Print and shaded views of the part. All mm, measured from the part's lowest x, y and z. A direction names the side the tool comes from. Round coordinates to 2 decimals unless told otherwise and drop trailing zeros. Order: outer loops, then holes, each group sorted by start corner. A loop starts at its lowest first (then second) coordinate and runs counter-clockwise, first axis right, second up. Notation, with made-up numbers: (34.5, 59) -> (70.5, 59) arc R9 cw to (70.5, 76) -> close; hole circle Ø5 at (-0.5, -36). An arc over 180 degrees is marked (long way). Answer as CSV lines item,"result".
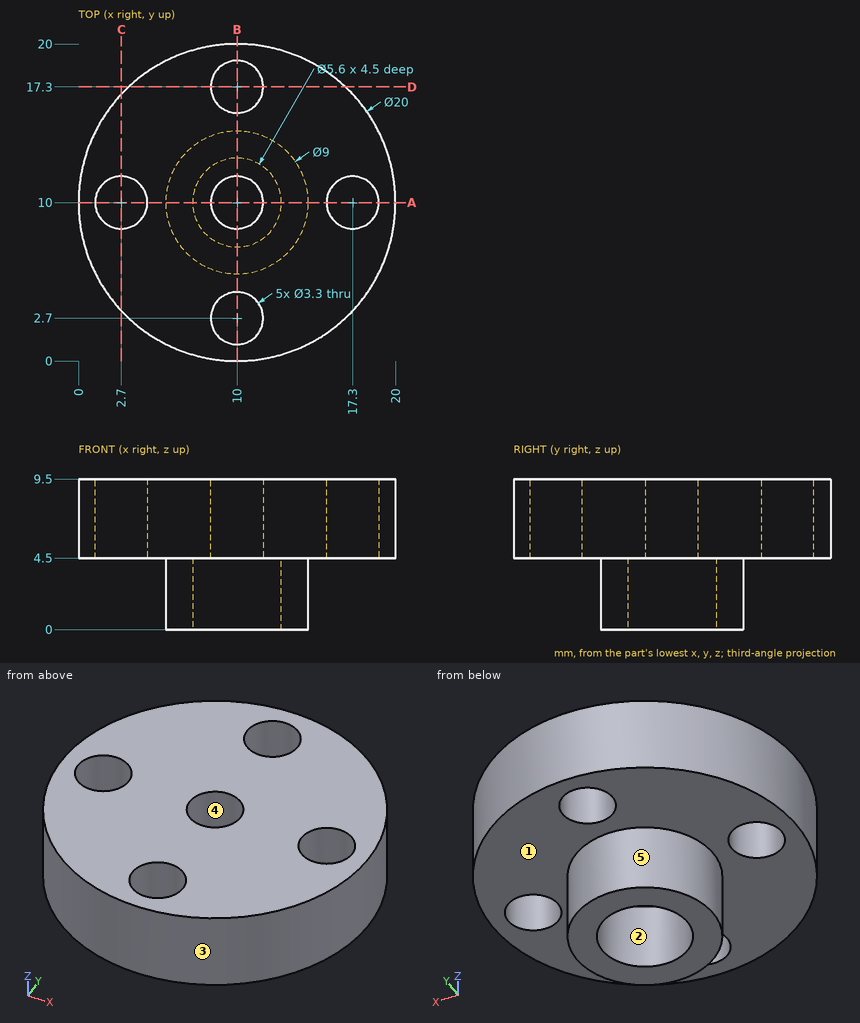
Q1. Tool access for the marked faces 4 and 5: list every direction of +Z, -Z, +X, -X, +Y, -Y with a clear straight run to the whole face (end or side of a thin tool).
Checks:
face 4,"+Z, -Z"
face 5,"-Z"
Q2. Mould opens along X. For the marked faces 1, 2 and 3 say: +X half, -X half, draft (parallel to the pull), parting line (faces both ways), or undercut.
Checks:
face 1,"draft"
face 2,"undercut"
face 3,"parting line"
Q3. Saw through at C-C (x = 2.7). Write the cut outline in (y, z), plus the area to 3 significant figures.
Checks:
outline,"(3.17, 4.5) -> (8.35, 4.5) -> (8.35, 9.5) -> (3.17, 9.5) -> close; (11.65, 4.5) -> (16.83, 4.5) -> (16.83, 9.5) -> (11.65, 9.5) -> close"
area,"51.8 mm²"
Q4. Flat gauge pins, fed straight in: pin 1 (1.7 mm diameter, centred on x = 9, y = 8.5, fed in from -Z); pin 2 (1.5 mm diameter, centred on x = 17.5, z = 5.5, fed in from -Y); pin 3 (3 mm diameter, centred on y = 3.5, z = 4.5, fed in from +X). Where does each tip first touch, or does it go through?
Checks:
pin 1,"z = 4.5"
pin 2,"y = 2.62"
pin 3,"x = 18.66"
Q5. Wall check: L1, parallel to Y at x = 10, z = 7.7; L2, parallel to Y at x = 10, z = 3.55; L3, parallel to X at y = 9.75, z = 5. Give the ranges that are in metal, low to high. Write a range as [from, to].
Checks:
L1,"[0, 1.05], [4.35, 8.35], [11.65, 15.65], [18.95, 20]"
L2,"[5.5, 7.2], [12.8, 14.5]"
L3,"[0, 1.07], [4.33, 8.37], [11.63, 15.67], [18.93, 20]"
Q6. Saw through at A-A (y = 10). Write the cut outline in (x, z).
Checks:
outline,"(0, 4.5) -> (1.05, 4.5) -> (1.05, 9.5) -> (0, 9.5) -> close; (4.35, 4.5) -> (5.5, 4.5) -> (5.5, 0) -> (7.2, 0) -> (7.2, 4.5) -> (8.35, 4.5) -> (8.35, 9.5) -> (4.35, 9.5) -> close; (11.65, 4.5) -> (12.8, 4.5) -> (12.8, 0) -> (14.5, 0) -> (14.5, 4.5) -> (15.65, 4.5) -> (15.65, 9.5) -> (11.65, 9.5) -> close; (18.95, 4.5) -> (20, 4.5) -> (20, 9.5) -> (18.95, 9.5) -> close"
